Input: part model. Units: mm. Frame: model coordinates. A direction names the side the tool comes from. Round coordinates to 2 decimals unless told otherwise and drop trailing zeros. Loops run counter-clockwise (first coordinate to the right, second up) from the corner with the lowest first, then second, coordinate; pieces in that order, holes last. Notation, with made-up numbers: (-39.75, -38) -> (-26.75, -38) arc R14 ccw to (-26.75, -31) -> close; hole circle Ø7 at (-27.5, 24.5). An arc over 180 degrees is marked (long way). Answer as a JSON object with one key per item and string values.
```python
from build123d import *

# Parameters (mm, degrees)
F0_W     = 10
F0_H     = 10
F0_R     = 1.65
F1_DEPTH = 30
F0_W_2   = 80
F0_H_2   = 80
F0_R_2   = 4.65
F0_W_3   = 33.5
F0_H_3   = 18.0101236328
F2_DEPTH = 2
F3_R     = 5
F4_SIZE  = 2
F5_W     = 34
F5_H     = 4
F6_DEPTH = 25


with BuildPart() as f1:
    # F0 (on Top) → F1 (new body)
    with BuildSketch(Plane.XY):
        with Locations((-0.4196270893, 17.7291296907)):
            Rectangle(F0_W, F0_H)
        with Locations((-0.4196270893, 17.7291296907)):
            Circle(F0_R, mode=Mode.SUBTRACT)
    extrude(amount=F1_DEPTH)



with BuildPart() as f1b:
    # F0 (on Top) → F1, piece 2 (new body)
    with BuildSketch(Plane.XY):
        with Locations((-0.4196270893, -15.7708703093)):
            Rectangle(F0_W, F0_H)
        with Locations((-0.4196270893, -15.7708703093)):
            Circle(F0_R, mode=Mode.SUBTRACT)
    extrude(amount=F1_DEPTH)


with BuildPart() as f1_1:
    add(f1.part)

    add(f1b.part)  # F2 merges F1b
    # F0 (on Top) → F2 (join)
    with BuildSketch(Plane.XY):
        with Locations((-0.4196270893, 0.9791296907)):
            Rectangle(F0_W_2, F0_H_2)
        with Locations((-32.9196270893, -31.5208703093)):
            Circle(F0_R_2, mode=Mode.SUBTRACT)
        with Locations((32.0803729107, -31.5208703093)):
            Circle(F0_R_2, mode=Mode.SUBTRACT)
        with Locations((-0.4196270893, -15.7708703093)):
            Rectangle(F0_W, F0_H, mode=Mode.SUBTRACT)
        with Locations((-32.9196270893, 33.4791296907)):
            Circle(F0_R_2, mode=Mode.SUBTRACT)
        with Locations((-0.4196270893, 0.9791296907)):
            Rectangle(F0_W_3, F0_H_3, mode=Mode.SUBTRACT)
        with Locations((-0.4196270893, 17.7291296907)):
            Rectangle(F0_W, F0_H, mode=Mode.SUBTRACT)
        with Locations((32.0803729107, 33.4791296907)):
            Circle(F0_R_2, mode=Mode.SUBTRACT)
    extrude(amount=F2_DEPTH)

    # F3
    f3_edges = [f1_1.edges().sort_by_distance(p)[0] for p in [
        (-40.419627, -39.02087, 1),
        (-40.419627, 40.97913, 1),
        (39.580373, -39.02087, 1),
        (39.580373, 40.97913, 1),
    ]]
    fillet(f3_edges, radius=F3_R)

    # F4
    f4_edges = [f1_1.edges().sort_by_distance(p)[0] for p in [
        (-0.419627, 22.72913, 2),
        (-0.419627, -10.77087, 2),
        (4.580373, -15.77087, 2),
        (4.580373, 17.72913, 2),
        (-0.419627, -20.77087, 2),
        (-0.419627, 12.72913, 2),
        (-5.419627, 17.72913, 2),
        (-5.419627, -15.77087, 2),
    ]]
    chamfer(f4_edges, length=F4_SIZE)

    # F5 (on face) → F6 (cut)
    with BuildSketch(Plane.XY.offset(2)):
        with BuildLine():
            Line((-20.4196270893, -16.5208703093), (-20.4196270893, 18.4791296907))
            ThreePointArc((-20.4196270893, 18.4791296907), (-21.8840931834, 22.0146635966), (-25.4196270893, 23.4791296907))
            ThreePointArc((-25.4196270893, 23.4791296907), (-28.9551609952, 22.0146635966), (-30.4196270893, 18.4791296907))
            Line((-30.4196270893, 18.4791296907), (-30.4196270893, -16.5208703093))
            ThreePointArc((-30.4196270893, -16.5208703093), (-28.9551609952, -20.0564042153), (-25.4196270893, -21.5208703093))
            ThreePointArc((-25.4196270893, -21.5208703093), (-21.8840931834, -20.0564042153), (-20.4196270893, -16.5208703093))
        make_face()
        with Locations((-0.4196270893, 32.9791296907)):
            Rectangle(F5_W, F5_H)
        with BuildLine():
            ThreePointArc((24.5803729107, 23.4791296907), (21.0448390048, 22.0146635966), (19.5803729107, 18.4791296907))
            Line((19.5803729107, 18.4791296907), (19.5803729107, -16.5208703093))
            ThreePointArc((19.5803729107, -16.5208703093), (21.0448390048, -20.0564042153), (24.5803729107, -21.5208703093))
            ThreePointArc((24.5803729107, -21.5208703093), (28.1159068166, -20.0564042153), (29.5803729107, -16.5208703093))
            Line((29.5803729107, -16.5208703093), (29.5803729107, 18.4791296907))
            ThreePointArc((29.5803729107, 18.4791296907), (28.1159068166, 22.0146635966), (24.5803729107, 23.4791296907))
        make_face()
        with Locations((-0.4196270893, -31.0208703093)):
            Rectangle(F5_W, F5_H)
    extrude(amount=-F6_DEPTH, mode=Mode.SUBTRACT)


solid = f1_1.part
```
1) Section C-C, the plane z = 10.25. Output: boundary loops of the cut face in (x, y), plus the area to 3 significant figures.
Output:
{"outline": "(-5.42, -20.77) -> (4.58, -20.77) -> (4.58, -10.77) -> (-5.42, -10.77) -> close; (-5.42, 12.73) -> (4.58, 12.73) -> (4.58, 22.73) -> (-5.42, 22.73) -> close; hole circle Ø3.3 at (-0.42, -15.77); hole circle Ø3.3 at (-0.42, 17.73)", "area": "183 mm^2"}
2) Section D-D, the plane x = -22. Output: boundary loops of the cut face in (y, z).
Output:
{"outline": "(-39.02, 0) -> (-20.17, 0) -> (-20.17, 2) -> (-39.02, 2) -> close; (22.13, 0) -> (40.98, 0) -> (40.98, 2) -> (22.13, 2) -> close"}
3) Ray query, probe 1 along X at (y, z) = (5.5, 1.75); probe 2 along X at (y, z) = (-34, 1.5); probe 3 along X at (y, z) = (-16, 12.5). Return the intervals inside material, ascending.
Output:
{"probe 1": "x = -40.42 to -30.42, -20.42 to -17.17, 16.33 to 19.58, 29.58 to 39.58", "probe 2": "x = -40.42 to -36.85, -28.99 to 28.15, 36.01 to 39.58", "probe 3": "x = -5.42 to -2.05, 1.21 to 4.58"}
4) Section A-A, the plane y = -12. Output: boundary loops of the cut face in (x, z), plus the area to 3 significant figures.
Output:
{"outline": "(-40.42, 0) -> (-30.42, 0) -> (-30.42, 2) -> (-40.42, 2) -> close; (-20.42, 0) -> (19.58, 0) -> (19.58, 2) -> (6.58, 2) -> (4.58, 4) -> (4.58, 30) -> (-5.42, 30) -> (-5.42, 4) -> (-7.42, 2) -> (-20.42, 2) -> close; (29.58, 0) -> (39.58, 0) -> (39.58, 2) -> (29.58, 2) -> close", "area": "404 mm^2"}
5) Contact query for flat-ended pins moving along their axis: P1, Ø8, axis at x = 2, z = 12, coming from the -Y side; P2, Ø3, axis at x = 0.5, z = 13.5, coming from the +Y side; P3, Ø10, axis at y = -7.5, z = 14, coming from the +X side. Output: stop coordinate, or through.
Output:
{"P1": "stops at y = -20.77", "P2": "stops at y = 22.73", "P3": "stops at x = 4.58"}
6) Section B-B, the plane x = 11. Output: boundary loops of the cut face in (y, z), plus the area to 3 significant figures.
Output:
{"outline": "(-39.02, 0) -> (-33.02, 0) -> (-33.02, 2) -> (-39.02, 2) -> close; (-29.02, 0) -> (-8.03, 0) -> (-8.03, 2) -> (-29.02, 2) -> close; (9.98, 0) -> (30.98, 0) -> (30.98, 2) -> (9.98, 2) -> close; (34.98, 0) -> (40.98, 0) -> (40.98, 2) -> (34.98, 2) -> close", "area": "108 mm^2"}
7) Reachability of faces 4 (the face through (-5.42, -16, 17)), 5 (the face through (-17.42, -31, 1)), 6 (the face through (39.58, 0, 1)), 7 (the face through (4.58, -16, 17)), 8 (the face through (-0.52, -9.78, 3.01)) from +Z, -Z, +X, -X, +Y, -Y: full face, straight path, thin tool, end or side. Return the list, or none.
Output:
{"face 4": "+Z, -X, +Y, -Y", "face 5": "+Z, -Z", "face 6": "+Z, -Z, +X, +Y, -Y", "face 7": "+Z, +X, +Y, -Y", "face 8": "+Z, +X, -X"}
8) Draft query along Y for faces 1 (the face through (-1, -39.021, 1)), 2 (the face through (-1, 10.4, 0)), 3 (the face through (-1, -29.021, 1)). Return one class per face: +Y half, -Y half, draft (parallel to the pull), parting line (faces both ways), or undercut.
Output:
{"face 1": "-Y half", "face 2": "draft", "face 3": "undercut"}
